Geometry check sheet. Reference: the model listing, model coordinates, mm. A direction names the side the tool comes from. Give positions to 0.01 mm unless a question says otherwise; leave off trailing zeros. Write each loop counter-clockwise with the first axis right and the second up, starting at its lowest first coordinate (ties: lowest second). Pieces come first, ordered by that corner, then holes. Notation, with made-up numbers: (-27, 56.5) -> (-3, 56.5) arc R11 cw to (-3, 68.5) -> close; hole circle Ø7 at (25.5, 42.25). An arc over 180 degrees is marked (long way). Write item = value, one per line. Start each with the question number.
1. Mould release check, pull along X, two halves, no side actions. Record for faces 1 (the cylindrical face through (-9.59, 6.26, 43.17)), 2 (the flat face through (-40, 0, -13)), 3 (the cylindrical face through (39.757, 6.887, -12.52)): pulls with the +X half, pulls with the -X half, needs draft (parallel to the pull), parting line crosses it, or undercut.
2. Cross-section at C-C, the plane y = 4.75. Record the cut outline in (x, z).
3. Set-up check for faces 4 (the flat face through (45, 26.67, 18)), 5 (the cylindrical face through (-10.41, 20.23, 46.89)), 6 (the flat face through (0, 12.7, 45)): record each of +Z, -Z, +X, -X, +Y, -Y from which the full face is reachable in a straight line by a thin tool's end or side.
4. Cross-section at A-A, the plane x = 0. Record the cut outline in (y, z).
5. Thickness scan on line 1 along Z through (x, y) = (0, 5.5); line 2 along X through (y, z) = (19.25, 0). Record the ranges inside material, lowest first.
6. Cross-section at B-B, the plane z = 0. Record the cut outline in (x, y), plus the area to 3 significant figures.
7. Cross-section at D-D, the plane y = 15.25. Record the cut outline in (x, z), plus the area to 3 significant figures.
8. Depth check by flat-ended pin: P1, Ø2, axis at y = 12.5, z = 19.5, coming from the -X side; P2, Ø5, axis at y = 23.5, z = 12.5, coming from the +X side; P3, Ø10, axis at x = 12.5, y = 23.5, coming from the +Z side. Enter the tip coordinate at first touch or a pass-through.
```python
from build123d import *

# Parameters (mm, degrees)
SKETCH1_R           = 44.2214
SKETCH1_R_2         = 41.6814
BOSS_EXTRUDE1_DEPTH = 12.7
SKETCH2_R           = 50.5714
SKETCH2_R_2         = 41.6814
BOSS_EXTRUDE2_DEPTH = 1.27
SKETCH3_R           = 50.5714
SKETCH3_R_2         = 48.0314
BOSS_EXTRUDE3_DEPTH = 12.7


with BuildPart() as part:
    # Sketch1 → Boss-Extrude1 (new body)
    with BuildSketch(Plane(origin=(0, 0, 0), x_dir=(1, 0, 0), z_dir=(0, 1, 0))):
        Circle(SKETCH1_R)
        Circle(SKETCH1_R_2, mode=Mode.SUBTRACT)
    extrude(amount=BOSS_EXTRUDE1_DEPTH)

    # Sketch2 → Boss-Extrude2 (add)
    with BuildSketch(Plane(origin=(0, 12.7, 0), x_dir=(1, 0, 0), z_dir=(0, 1, 0))):
        Circle(SKETCH2_R)
        Circle(SKETCH2_R_2, mode=Mode.SUBTRACT)
    extrude(amount=BOSS_EXTRUDE2_DEPTH)

    # Sketch3 → Boss-Extrude3 (add)
    with BuildSketch(Plane(origin=(0, 13.97, 0), x_dir=(1, 0, 0), z_dir=(0, 1, 0))):
        Circle(SKETCH3_R)
        Circle(SKETCH3_R_2, mode=Mode.SUBTRACT)
    extrude(amount=BOSS_EXTRUDE3_DEPTH)


solid = part.part
```
Answers:
q1.face_1 = parting line crosses it
q1.face_2 = needs draft
q1.face_3 = undercut
q2.outline = circle Ø88.44 at (0, 0); hole circle Ø83.36 at (0, 0)
q3.face_4 = +Z, -Z, +X, -X, +Y
q3.face_5 = +Y
q3.face_6 = -Y
q4.outline = (0, -44.22) -> (12.7, -44.22) -> (12.7, -50.57) -> (26.67, -50.57) -> (26.67, -48.03) -> (13.97, -48.03) -> (13.97, -41.68) -> (0, -41.68) -> close; (0, 41.68) -> (13.97, 41.68) -> (13.97, 48.03) -> (26.67, 48.03) -> (26.67, 50.57) -> (12.7, 50.57) -> (12.7, 44.22) -> (0, 44.22) -> close
q5.line_1 = -44.22 to -41.68, 41.68 to 44.22
q5.line_2 = -50.57 to -48.03, 48.03 to 50.57
q6.outline = (-50.57, 12.7) -> (-44.22, 12.7) -> (-44.22, 0) -> (-41.68, 0) -> (-41.68, 13.97) -> (-48.03, 13.97) -> (-48.03, 26.67) -> (-50.57, 26.67) -> close; (41.68, 0) -> (44.22, 0) -> (44.22, 12.7) -> (50.57, 12.7) -> (50.57, 26.67) -> (48.03, 26.67) -> (48.03, 13.97) -> (41.68, 13.97) -> close
q6.area = 152 mm^2
q7.outline = circle Ø101.14 at (0, 0); hole circle Ø96.06 at (0, 0)
q7.area = 787 mm^2
q8.P1 = -47.06
q8.P2 = 49.57
q8.P3 = 50.01
